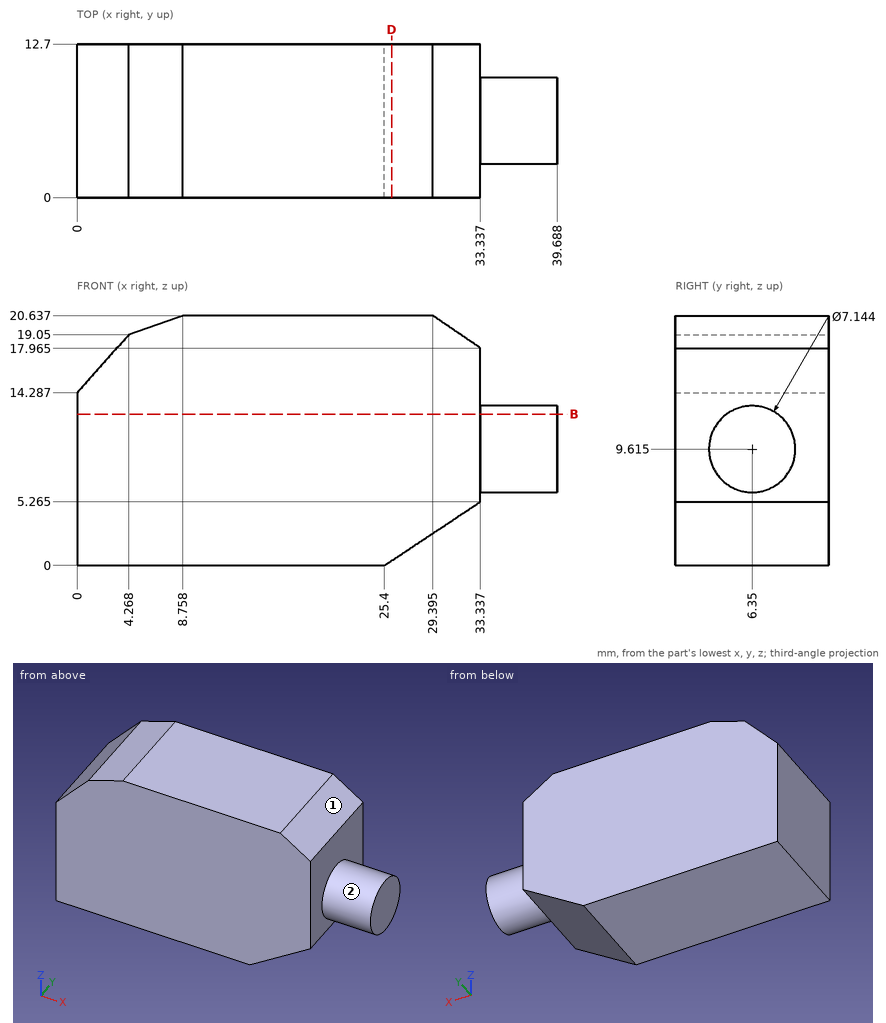
The figure shows three views and two pictorial views of one solid part (mm, origin at its lowest corner). Answer the questions. A direction names the side the tool comes from. Coordinates: 2 decimals unless noted, no trailing zeros. Loops run counter-clockwise (first coordinate to the right, second up) from the corner with the lowest first, then second, coordinate; pieces in that order, holes last. Notation, with made-up numbers: M 24,38 L 29,38 A21 ccw 29,76 Z; hole C -37,16 d2. An arc over 180 degrees is marked long. Use CSV: the item, a comma, the result in double quotes. Start each with the question number.
(1) Find section B-B, the plane z = 12.5. Give the vertices of the cut face in (x, y) (1 decimal), then the cut area to 3 significant figures.
(2) Find section D-D, the plane x = 26. Give the vertices of the cut face in (y, z).
(3) Consider line 1 (X direction, y = 2.5, z = 10); line 2 (Z direction, x = 31.5, y = 1.75) (1 decimal); line 3 (Z direction, x = 26, y = 2). Determine where each line is inside the solid, lowest interval first.
(4) Given pin 1 Ø1 at (y, z) = (8.5, 17) entering from -X; pin 2 Ø1.5 at (x, y) = (33.5, 8.5) entering from +Z; pin 3 Ø1 at (y, z) = (2.5, 18.5) entering from -X (1 decimal), each flat-ended and moving along its own axis, determine where each tip first touches the part or whether it passes through.
(5) For the marked faces 1 and 2, determine the directions among +Z, -Z, +X, -X, +Y, -Y from which every point of the face is accessible in a straight line to the end or side of a thin tool.
Recorded:
1,outline,"M 0,0 L 33.3,0 L 33.3,4.2 L 39.7,4.2 L 39.7,8.5 L 33.3,8.5 L 33.3,12.7 L 0,12.7 Z"
1,area,"450 mm^2"
2,outline,"M 0,0.4 L 12.7,0.4 L 12.7,20.64 L 0,20.64 Z"
3,line 1,"x = 0 to 33.34"
3,line 2,"z = 4 to 19.2"
3,line 3,"z = 0.4 to 20.64"
4,pin 1,"stops at x = 1.98"
4,pin 2,"stops at z = 18.36"
4,pin 3,"stops at x = 3.3"
5,face 1,"+Z, +X, +Y, -Y"
5,face 2,"+X"
